The model under review builds one solid part; all positions refer to its coordinate system, in mm. A direction names the side the tool comes from. Give positions to 0.01 mm unless a question says otherwise; leave off trailing zeros. Loops run counter-clockwise (first coordinate to the right, second up) from the corner with the lowest first, then second, coordinate; pieces in that order, holes last. Notation, with made-up numbers: M -37.75,-31.75 L -2.75,-31.75 A29 cw -2.75,-7.75 Z; hole C 26.25,-10.75 d8. An arc over 180 degrees is marked long. Put each result on its own line as item: value. Start each with the question number.
Autodesk Inventor part; units mm, degrees
ref_plane "YZ Plane" through (0, 0, 0) normal (1, 0, 0) x (0, 1, 0)
ref_plane "XZ Plane" through (0, 0, 0) normal (0, 1, 0) x (-1, 0, 0)
ref_plane "XY Plane" through (0, 0, 0) normal (0, 0, 1) x (1, 0, 0)
sketch "Sketch1" plane through (0, 0, 0) normal (0, 1, 0) x (-1, 0, 0)
  line L0 (0, 0) -> (101.6, 0)
  line L1 (101.6, 0) -> (101.6, 50.8)
  line L2 (101.6, 50.8) -> (0, 50.8)
  line L3 (0, 50.8) -> (0, 0)
  line L4 (101.6, 0) -> (20.6375, 0)
  line L5 (20.6375, 50.8) -> (101.6, 50.8)
  line L6 (101.6, 50.8) -> (101.6, 0)
  line L7 (20.6375, 0) -> (0, 0)
  line L8 (0, 0) -> (0, 12.7)
  line L9 (0, 12.7) -> (20.6375, 12.7)
  line L10 (20.6375, 12.7) -> (20.6375, 0)
  line L11 (20.6375, 50.8) -> (0, 50.8)
  line L12 (0, 50.8) -> (0, 38.1)
  line L13 (0, 38.1) -> (20.6375, 38.1)
  line L14 (20.6375, 38.1) -> (20.6375, 50.8)
  line L15 (96.8375, 0) -> (84.1375, 0)
  line L16 (84.1375, 0) -> (84.1375, 3.175)
  line L17 (84.1375, 3.175) -> (96.8375, 3.175)
  line L18 (96.8375, 3.175) -> (96.8375, 0)
  line L19 (71.4375, 0) -> (58.7375, 0)
  line L20 (58.7375, 0) -> (58.7375, 3.175)
  line L21 (58.7375, 3.175) -> (71.4375, 3.175)
  line L22 (71.4375, 3.175) -> (71.4375, 0)
  line L23 (46.0375, 0) -> (33.3375, 0)
  line L24 (33.3375, 0) -> (33.3375, 3.175)
  line L25 (33.3375, 3.175) -> (46.0375, 3.175)
  line L26 (46.0375, 3.175) -> (46.0375, 0)
  line L27 (96.8375, 50.8) -> (84.1375, 50.8)
  line L28 (84.1375, 50.8) -> (84.1375, 47.625)
  line L29 (84.1375, 47.625) -> (96.8375, 47.625)
  line L30 (96.8375, 47.625) -> (96.8375, 50.8)
  line L31 (71.4375, 50.8) -> (58.7375, 50.8)
  line L32 (58.7375, 50.8) -> (58.7375, 47.625)
  line L33 (58.7375, 47.625) -> (71.4375, 47.625)
  line L34 (71.4375, 47.625) -> (71.4375, 50.8)
  line L35 (101.6, 38.1) -> (98.425, 38.1)
  line L36 (98.425, 38.1) -> (98.425, 31.75)
  line L37 (98.425, 31.75) -> (101.6, 31.75)
  line L38 (101.6, 31.75) -> (101.6, 38.1)
  line L39 (101.6, 19.05) -> (98.425, 19.05)
  line L40 (98.425, 19.05) -> (98.425, 12.7)
  line L41 (98.425, 12.7) -> (101.6, 12.7)
  line L42 (101.6, 12.7) -> (101.6, 19.05)
  line L43 (46.0375, 50.8) -> (46.0375, 47.625)
  line L44 (46.0375, 47.625) -> (33.3375, 47.625)
  line L45 (33.3375, 47.625) -> (33.3375, 50.8)
  line L46 (33.3375, 50.8) -> (46.0375, 50.8)
  line L47 (26.9875, 0) -> (52.3875, 0)
  line L48 (52.3875, 0) -> (52.3875, -19.05)
  line L49 (52.3875, -19.05) -> (26.9875, -19.05)
  line L50 (26.9875, -19.05) -> (26.9875, 0)
  line L51 (26.9875, 50.8) -> (26.9875, 69.85)
  line L52 (26.9875, 69.85) -> (52.3875, 69.85)
  line L53 (52.3875, 69.85) -> (52.3875, 50.8)
  line L54 (52.3875, 50.8) -> (26.9875, 50.8)
  circle A0 centre (39.6875, -9.525) radius 3.302
  circle A1 centre (39.6875, 60.325) radius 3.302
  line L55 (0, 19.05) -> (0, 31.75)
  line L56 (0, 31.75) -> (-50.8, 31.75)
  line L57 (-50.8, 31.75) -> (-50.8, 19.05)
  line L58 (-50.8, 19.05) -> (0, 19.05)
  circle A2 centre (-43.5387, 25.4) radius 3.302
  line L59 (26.9875, 50.8) -> (24.8905, 50.8)
  line L60 (26.9875, 0) -> (25.4, 0)
  line L61 (20.6375, 0) -> (17.4625, 0)
  line L62 (17.4625, 0) -> (17.4625, 3.175)
  line L63 (17.4625, 3.175) -> (20.6375, 3.175)
  line L64 (20.6375, 3.175) -> (20.6375, 0)
  line L65 (20.6375, 50.8) -> (17.4625, 50.8)
  line L66 (17.4625, 50.8) -> (17.4625, 47.625)
  line L67 (17.4625, 47.625) -> (20.6375, 47.625)
  line L68 (20.6375, 47.625) -> (20.6375, 50.8)
  line L69 (20.6375, 0) -> (-11.1125, 0)
  line L70 (-11.1125, 0) -> (-11.1125, 50.8)
  line L71 (-11.1125, 50.8) -> (20.6375, 50.8)
  line L72 (20.6375, 50.8) -> (20.6375, 0)
  point P0 (96.8375, 0)
  point P1 (96.8375, 50.8)
  point P2 (84.1375, 50.8)
  point P3 (71.4375, 50.8)
  point P4 (58.7375, 50.8)
  point P5 (46.0375, 50.8)
  point P6 (33.3375, 50.8)
  point P7 (33.3375, 0)
  point P8 (46.0375, 0)
  point P9 (58.7375, 0)
  point P10 (71.4375, 0)
  point P11 (84.1375, 0)
  point P12 (26.9875, 0)
  point P13 (52.3875, 0)
  point P14 (52.3875, 50.8)
  point P15 (26.9875, 50.8)
  point P16 (17.4625, 0)
  point P17 (0, 50.8)
  point P18 (-11.1125, 31.75)
  point P19 (-11.1125, 19.05)
  dimension "d56" = 101.6
  dimension "d57" = 50.8
  dimension "d59" = 50.8
  dimension "d60" = 12.7
  dimension "d61" = 12.7
  dimension "d62" = 12.7
  dimension "d63" = 3.175
  dimension "d64" = 12.7
  dimension "d65" = 3.175
  dimension "d66" = 12.7
  dimension "d67" = 4.7625
  dimension "d68" = 12.7
  dimension "d69" = 3.175
  dimension "d70" = 12.7
  dimension "d71" = 12.7
  dimension "d72" = 3.175
  dimension "d73" = 12.7
  dimension "d74" = 3.175
  dimension "d77" = 4.7625
  dimension "d78" = 12.7
  dimension "d79" = 3.175
  dimension "d80" = 6.35
  dimension "d81" = 12.7
  dimension "d82" = 3.175
  dimension "d83" = 6.35
  dimension "d84" = 12.7
  dimension "d86" = 44.45
  dimension "d89" = 3.175
  dimension "d90" = 12.7
  dimension "d91" = 12.7
  dimension "d94" = 25.4
  dimension "d99" = 25.4
  dimension "d116" = 6.604
  dimension "d117" = 9.525
  dimension "d118" = 6.604
  dimension "d119" = 9.525
  dimension "d122" = 9.525
  dimension "d123" = 9.525
  dimension "d128" = 12.7
  dimension "d129" = 50.8
  dimension "d130" = 6.604
  dimension "d131" = 6.35
  dimension "d132" = 12.7
  dimension "d134" = 12.7
  dimension "d141" = 25.4
  dimension "d144" = 6.35
  dimension "d145" = 6.35
  dimension "d147" = 3.175
  dimension "d148" = 3.175
  dimension "d149" = 3.175
  dimension "d150" = 3.175
  dimension "d151" = 12.7
  dimension "d152" = 12.7
  dimension "d155" = 31.75
extrude "Extrusion10" add sketch "Sketch1" along normal blind 25.4 contours L3 L9 L10 L63 L62 L0 | L69 L70 L58 L3 | L3 L13 L72 L9 | L10 L72 L14 L2 L45 L44 L43 L32 L33 L34 L28 L29 L30 L1 L35 L36 L37 L39 L40 L41 L0 L18 L17 L16 L22 L21 L20 L26 L25 L24 | L58 L70 L56 L3 | L58 L57 L56 L70 | L56 L70 L71 L3 | L13 L3 L2 L66 L67 L14 | L0 L48 L49 L50 | L51 L52 L53 L2
equation "\"BendRadius\" = Thickness"
equation "\"BendReliefWidth\" = Thickness"
equation "\"BendReliefDepth\" = 0.5 * Thickness"
equation "\"CornerReliefSize\" = 4 * Thickness"
equation "\"MinimumRemnant\" = 2 * Thickness"
equation "\"TransitionRadius\" = BendRadius"
equation "\"JacobiRadiusSize\" = BendRadius"
equation "\"GapSize\" = Thickness"
properties part number "v8_Burrow_Base_Detachable_EXT_LICK_SPOUT"
(1) We need section C-C, the plane y = 2.5. State how many separate pieces and enclosed holes the cut face has, plus the area to 3 significant figures.
(2) Draft analysis for pull direction Z (two halves, no side actions). For faces 6 (the flat face through (-40, 13, 0)), 7 (the flat face through (-40, 13, -19.05)), 8 (the flat face through (-99, 13, 50.8)), state which applies: +Z half, -Z half, draft (parallel to the pull), parting line (faces both ways), or undercut.
(3) For faces 1 (the flat face through (-26.988, 13, 60)), 2 (the flat face through (-17.462, 13, 49)), 3 (the flat face through (-100, 13, 12.7)), 4 (the flat face through (-40, 13, 47.625)), 5 (the flat face through (-78, 13, 50.8)), list the 3-axis set-ups (+Z, -Z, +X, -X, +Y, -Y) from which the entire face can be reached by the end or side of a thin tool; tool diameter is ignored.
(4) To check wall thickness, follow L1, parallel to Z at x = -21, y = 15.25; L2, parallel to X at y = 19, z = 35 (1 decimal); L3, parallel to Z at x = -66.5, y = 12 (3 decimals). State the ranges of each line that lie inside material, in increasing order. Write a range as [from, to].
(5) We need section A-A, the plane z = 25.4. Write out the cut boundary in (x, y), plus the area to 3 significant figures.
(6) Insertion check: pin 1 (7.5 mm diameter, centred on x = -1.5, y = 9.5, fed in from +Z); pin 2 (3.5 mm diameter, centred on y = 8, z = 2, fed in from +X); pin 3 (4 mm diameter, centred on x = -8.5, y = 14, fed in from -Z). Each pin has a flat end and moves straight along its axis. Give the tip position at first contact, or say it passes through.
(7) We need section B-B, the plane x = -10.5. Write out the cut boundary in (y, z), plus the area to 3 significant figures.
Check sheet entries:
1. separate pieces: 1
1. enclosed holes: 5
1. area: 6,790 mm²
2. face 6: undercut
2. face 7: -Z half
2. face 8: +Z half
3. face 1: +Z, +X, +Y, -Y
3. face 2: +Z, +Y, -Y
3. face 3: -X, +Y, -Y
3. face 4: +Y, -Y
3. face 5: +Z, -X, +Y, -Y
4. L1: z = [0, 50.8]
4. L2: x = [-98.4, 11.1]
4. L3: z = [3.175, 47.625]
5. outline: M -101.6,0 L 40.24,0 L 40.24,25.4 L -101.6,25.4 Z; M 46.84,0 L 50.8,0 L 50.8,25.4 L 46.84,25.4 Z
5. area: 3,700 mm²
6. pin 1: stops at z = 50.8
6. pin 2: stops at x = 11.11
6. pin 3: stops at z = 0
7. outline: M 0,0 L 25.4,0 L 25.4,50.8 L 0,50.8 Z
7. area: 1,290 mm²
